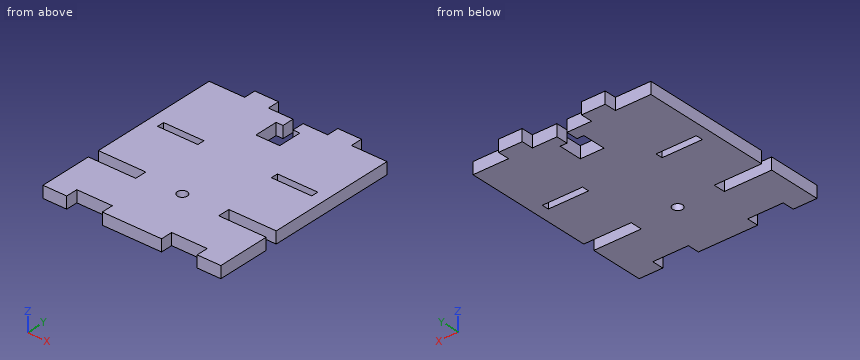
from build123d import *

# Parameters (mm, degrees)
SKETCH1_W           = 75
SKETCH1_H           = 17.5
SKETCH1_R           = 2.1
SKETCH1_W_2         = 10
SKETCH1_H_2         = 5
SKETCH1_W_3         = 25
BOSS_EXTRUDE1_DEPTH = 5
SKETCH2_W           = 75
SKETCH2_H           = 55
BOSS_EXTRUDE2_DEPTH = 5
SKETCH3_W           = 10
SKETCH3_H           = 5
BOSS_EXTRUDE3_DEPTH = 5
SKETCH4_W           = 4.2
SKETCH4_H           = 5
SKETCH4_H_2         = 3.2
SKETCH4_H_3         = 1.8
SKETCH4_W_2         = 1.4
CUT_EXTRUDE1_DEPTH  = 5
SKETCH5_W           = 10
SKETCH5_H           = 10
CUT_EXTRUDE2_DEPTH  = 5
SKETCH6_W           = 17.000000092
SKETCH6_H           = 3
CUT_EXTRUDE3_DEPTH  = 10


with BuildPart() as part:
    # Sketch1 → Boss-Extrude1 (new body)
    with BuildSketch(Plane.XY):
        with Locations((37.5, 8.75)):
            Rectangle(SKETCH1_W, SKETCH1_H)
        Polygon((20, 22.5), (20, 17.5), (55, 17.5), (55, 22.5), (41.830127019, 22.5), (33.169872981, 22.5), align=None)
        with Locations((37.5, 20)):
            Circle(SKETCH1_R, mode=Mode.SUBTRACT)
        with BuildLine():
            ThreePointArc((41.830127019, 22.5), (37.5, 25), (33.169872981, 22.5))
            Line((33.169872981, 22.5), (41.830127019, 22.5))
        make_face()
        Polygon((0, 17.5), (0, 0), (10, 0), (25, 0), (50, 0), (65, 0), (75, 0), (75, 17.5), (55, 17.5), (20, 17.5), align=None)
        with Locations((70, -2.5)):
            Rectangle(SKETCH1_W_2, SKETCH1_H_2)
        with Locations((37.5, -2.5)):
            Rectangle(SKETCH1_W_3, SKETCH1_H_2)
        with Locations((5, -2.5)):
            Rectangle(SKETCH1_W_2, SKETCH1_H_2)
    extrude(amount=BOSS_EXTRUDE1_DEPTH)

    # Sketch2 → Boss-Extrude2 (add)
    with BuildSketch(Plane(origin=(0, 0, 0), x_dir=(-1, 0, 0), z_dir=(0, 0, -1))):
        with Locations((-37.5, 50)):
            Rectangle(SKETCH2_W, SKETCH2_H)
    extrude(amount=-BOSS_EXTRUDE2_DEPTH)

    # Sketch3 → Boss-Extrude3 (add)
    with BuildSketch(Plane(origin=(0, 0, 0), x_dir=(-1, 0, 0), z_dir=(0, 0, -1))):
        with Locations((-55, 80)):
            Rectangle(SKETCH3_W, SKETCH3_H)
        with Locations((-20, 80)):
            Rectangle(SKETCH3_W, SKETCH3_H)
    extrude(amount=-BOSS_EXTRUDE3_DEPTH)

    # Sketch4 → Cut-Extrude1 (cut)
    with BuildSketch(Plane(origin=(0, 0, 0), x_dir=(-1, 0, 0), z_dir=(0, 0, -1))):
        with Locations((-37.5, 75)):
            Rectangle(SKETCH4_W, SKETCH4_H)
        with Locations((-37.5, 70.9)):
            Rectangle(SKETCH4_W, SKETCH4_H_2)
        with Locations((-37.5, 68.4)):
            Rectangle(SKETCH4_W, SKETCH4_H_3)
        with Locations((-40.3, 70.9)):
            Rectangle(SKETCH4_W_2, SKETCH4_H_2)
        with Locations((-34.7, 70.9)):
            Rectangle(SKETCH4_W_2, SKETCH4_H_2)
    extrude(amount=-CUT_EXTRUDE1_DEPTH, mode=Mode.SUBTRACT)

    # Sketch5 → Cut-Extrude2 (cut)
    with BuildSketch(Plane(origin=(0, 0, 0), x_dir=(-1, 0, 0), z_dir=(0, 0, -1))):
        with Locations((-37.5, 67.5)):
            Rectangle(SKETCH5_W, SKETCH5_H)
    extrude(amount=-CUT_EXTRUDE2_DEPTH, mode=Mode.SUBTRACT)

    # Sketch6 → Cut-Extrude3 (cut)
    with BuildSketch(Plane(origin=(0, 0, 0), x_dir=(-1, 0, 0), z_dir=(0, 0, -1))):
        with Locations((-61.499999954, 47.499999965)):
            Rectangle(SKETCH6_W, SKETCH6_H)
        with Locations((-13.500000046, 47.499999965)):
            Rectangle(SKETCH6_W, SKETCH6_H)
    extrude(amount=-CUT_EXTRUDE3_DEPTH, mode=Mode.SUBTRACT)


solid = part.part
Can you work these out from the model? Positions are in its coordinate system, mm. Give positions to 0.01 mm unless a question says otherwise; leave off trailing zeros. Loops run counter-clockwise (first coordinate to the right, second up) from the corner with the lowest first, then second, coordinate; pieces in that order, holes last. Notation, with made-up numbers: (29.25, -37) -> (48.25, -37) arc R29 ccw to (48.25, -11) -> close; hole circle Ø10 at (88, -3). An arc over 180 degrees is marked (long way). Write item = value, one per line.
1) Suppose I cut it at A-A on x = 37.5. Write out the boundary of the cut face in (y, z).
Check result:
outline = (-5, 0) -> (17.9, 0) -> (17.9, 5) -> (-5, 5) -> close; (22.1, 0) -> (62.5, 0) -> (62.5, 5) -> (22.1, 5) -> close
2) Suppose I cut it at C-C on x = 57.5. Write out the boundary of the cut face in (y, z), then the cut area to 4 significant figures.
Check result:
outline = (0, 0) -> (17.5, 0) -> (17.5, 5) -> (0, 5) -> close; (22.5, 0) -> (46, 0) -> (46, 5) -> (22.5, 5) -> close; (49, 0) -> (82.5, 0) -> (82.5, 5) -> (49, 5) -> close
area = 372.5 mm2
3) I need wall thicknesses on L1, parallel to Y at x = 66, z = 1.75; L2, parallel to Y at x = 17.5, z = 1.6; L3, parallel to Y at x = 37.5, z = 3.1. Which ranges of each line are inside material? Lowest first, please. Write a range as from..to.
Check result:
L1 = -5..17.5, 22.5..46, 49..77.5
L2 = 0..17.5, 22.5..46, 49..82.5
L3 = -5..17.9, 22.1..62.5
4) Suppose I cut it at B-B on y = 20. Write out the boundary of the cut face in (x, z).
Check result:
outline = (20, 0) -> (35.4, 0) -> (35.4, 5) -> (20, 5) -> close; (39.6, 0) -> (55, 0) -> (55, 5) -> (39.6, 5) -> close
5) Will these pins go through, and if not, where does the flat tip stop? pin 1 (1.5 mm diameter, centred on x = 54, z = 1.5, fed in from -Y); pin 2 (1 mm diameter, centred on y = 16, z = 1.5, fed in from -X); pin 3 (2.5 mm diameter, centred on y = 21, z = 2, fed in from +X).
Check result:
pin_1 = 0
pin_2 = 0
pin_3 = 55
6) Suppose I cut it at D-D on z = 3.1. Give the number of separate pieces and of enclosed holes in the cut face, then the cut area to 3 significant figures.
Check result:
separate_pieces = 1
enclosed_holes = 3
area = 5,700 mm2
